The drawing under review shows one solid part. Ordinate dimensions are in mm from its lowest x, y, z. Round coordinates to 2 decimals unless told otherwise and drop trailing zeros. Write each loop counter-clockwise with the first axis right and the second up, starting at its lowest first coordinate (ties: lowest second). Pieces come first, ordered by that corner, then holes. Notation, with made-up numbers: (48.25, 56.5) -> (59.25, 56.5) arc R8 ccw to (59.25, 62.5) -> close; hole circle Ø5 at (3.5, 37). An arc over 180 degrees is marked (long way). Answer in a Markdown table with one row per item.
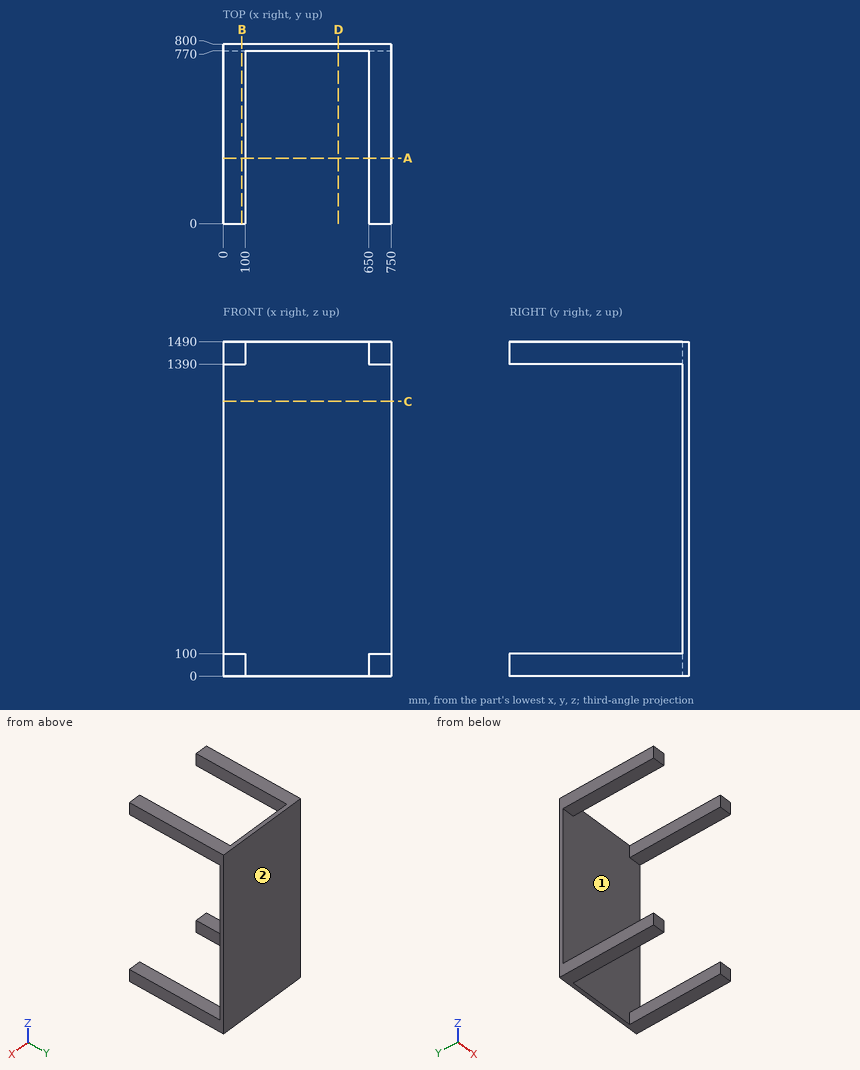
1) Consider section A-A on y = 291. State the section outline as (x, z) points.
Solved:
| item | result |
|---|---|
| outline | (0, 0) -> (100, 0) -> (100, 100) -> (0, 100) -> close; (0, 1390) -> (100, 1390) -> (100, 1490) -> (0, 1490) -> close; (650, 0) -> (750, 0) -> (750, 100) -> (650, 100) -> close; (650, 1390) -> (750, 1390) -> (750, 1490) -> (650, 1490) -> close |
2) Consider section D-D on x = 514. State the section outline as (y, z) points, then the cut area to 3 significant figures.
Solved:
| item | result |
|---|---|
| outline | (770, 0) -> (800, 0) -> (800, 1490) -> (770, 1490) -> close |
| area | 44,700 mm² |
3) Mouldability with a two-part tool opening along Z and no side actions: class the marked faces 1 and 2 as pulls with the +Z half, pulls with the -Z half, needs draft (parallel to the pull), parting line crosses it, or undercut.
Solved:
| item | result |
|---|---|
| face 1 | undercut |
| face 2 | needs draft |
4) Consider section C-C on z = 1224. State the section outline as (x, y) points.
Solved:
| item | result |
|---|---|
| outline | (0, 770) -> (750, 770) -> (750, 800) -> (0, 800) -> close |
5) For line 1 (Z direction, x = 702, y = 310); line 2 (Y direction, x = 535, z = 1087), list the stretches that pass through material, from the lowest coordinate up. Write a range as [from, to].
Solved:
| item | result |
|---|---|
| line 1 | [0, 100], [1390, 1490] |
| line 2 | [770, 800] |
6) Consider section B-B on x = 84. State the section outline as (y, z) points, then the cut area to 3 significant figures.
Solved:
| item | result |
|---|---|
| outline | (0, 0) -> (800, 0) -> (800, 1490) -> (0, 1490) -> (0, 1390) -> (770, 1390) -> (770, 100) -> (0, 100) -> close |
| area | 199,000 mm² |
7) Clearance check with a flat-ended pin moving along its axis: pin 1 Ø6 at (x, z) = (639, 666) entering from -Y. State where the tip first meets the part, or that it passes through.
Solved:
| item | result |
|---|---|
| pin 1 | y = 770 |
